Design review of the part built by this model. Coordinates are the model's own, in mm. A direction names the side the tool comes from. Round coordinates to 2 decimals unless told otherwise and drop trailing zeros. Order: outer loops, then holes, each group sorted by start corner. A loop starts at its lowest first (then second) coordinate and runs counter-clockwise, first axis right, second up. Notation, with made-up numbers: (29, 78) - (76, 78) arc R18 cw to (76, 88) - close; hole circle Ø8 at (22, 80). An arc over 180 degrees is marked (long way). Write item = value, one per line.
from build123d import *

# Parameters (mm, degrees)
SKETCH_1_R          = 12.25
SKETCH_1_R_2        = 5.5
SKETCH_1_R_3        = 1.25
EXTRUDE_1_DEPTH     = 3.5
SKETCH_2_R          = 2.25
CUT_EXTRUDE_1_DEPTH = 2
CHAMFER_1_SIZE      = 1


with BuildPart() as part:
    # Эскиз1 → Бобышка-Вытянуть1 (new body)
    with BuildSketch(Plane(origin=(0, 0, 0), x_dir=(1, 0, 0), z_dir=(0, 1, 0))):
        with Locations(Location((0, 0, 0), (0, 0, 270))):
            Circle(SKETCH_1_R)
        with Locations(Location((0, 0, 0), (0, 0, 270))):
            Circle(SKETCH_1_R_2, mode=Mode.SUBTRACT)
        with Locations(Location((0, 9.5, 0), (0, 0, 270))):
            Circle(SKETCH_1_R_3, mode=Mode.SUBTRACT)
        with Locations(Location((9.5, 0, 0), (0, 0, 270))):
            Circle(SKETCH_1_R_3, mode=Mode.SUBTRACT)
        with Locations(Location((0, -9.5, 0), (0, 0, 270))):
            Circle(SKETCH_1_R_3, mode=Mode.SUBTRACT)
        with Locations(Location((-9.5, 0, 0), (0, 0, 270))):
            Circle(SKETCH_1_R_3, mode=Mode.SUBTRACT)
    extrude(amount=EXTRUDE_1_DEPTH)

    # Эскиз2 → Вырез-Вытянуть1 (cut)
    with BuildSketch(Plane(origin=(0, 3.5, 0), x_dir=(1, 0, 0), z_dir=(0, 1, 0))):
        with Locations(Location((0, 9.5, 0), (0, 0, 270))):
            Circle(SKETCH_2_R)
        with Locations(Location((9.5, 0, 0), (0, 0, 270))):
            Circle(SKETCH_2_R)
        with Locations(Location((0, -9.5, 0), (0, 0, 270))):
            Circle(SKETCH_2_R)
        with Locations(Location((-9.5, 0, 0), (0, 0, 270))):
            Circle(SKETCH_2_R)
    extrude(amount=-CUT_EXTRUDE_1_DEPTH, mode=Mode.SUBTRACT)

    # Фаска1
    chamfer_1_edges = [part.edges().sort_by_distance(p)[0] for p in [
        (0, 3.5, -5.5),
    ]]
    chamfer(chamfer_1_edges, length=CHAMFER_1_SIZE)


solid = part.part
1) The part is to be moulded in two halves that separate along Z. For faces 3 (the cylindrical face through (10.74, 0.74, -0.16)), 4 (the cylindrical face through (3.68, 1.726, 11.684)), 5 (the flat face through (0, 0, -6)), say which applies: released by +Z, released by -Z, zero draft, split by the parting line, or undercut.
Findings:
face_3 = undercut
face_4 = split by the parting line
face_5 = zero draft
2) We need section A-A on x = 0. Write out the cut boundary in (y, z).
Findings:
outline = (0, -12.25) - (3.5, -12.25) - (3.5, -11.75) - (1.5, -11.75) - (1.5, -10.75) - (0, -10.75) - close; (0, -8.25) - (1.5, -8.25) - (1.5, -7.25) - (3.5, -7.25) - (3.5, -6.5) - (2.5, -5.5) - (0, -5.5) - close; (0, 5.5) - (2.5, 5.5) - (3.5, 6.5) - (3.5, 7.25) - (1.5, 7.25) - (1.5, 8.25) - (0, 8.25) - close; (0, 10.75) - (1.5, 10.75) - (1.5, 11.75) - (3.5, 11.75) - (3.5, 12.25) - (0, 12.25) - close
3) For faces 1 (the cylindrical face through (11.73, 2.51, -0.29)), 2 (the flat face through (-5, 3.5, 5)), list the 3-axis set-ups (+Z, -Z, +X, -X, +Y, -Y) from which the entire face can be reached by the end or side of a thin tool; tool diameter is ignored.
Findings:
face_1 = +Y
face_2 = +Z, -Z, +X, -X, +Y
4) We need section C-C on y = 1.85. Write out the cut boundary in (x, z).
Findings:
outline = circle Ø24.5 at (0, 0); hole circle Ø4.5 at (-9.5, 0); hole circle Ø11 at (0, 0); hole circle Ø4.5 at (0, -9.5); hole circle Ø4.5 at (0, 9.5); hole circle Ø4.5 at (9.5, 0)
5) Clearance check with flat-ended pins moving along their axes: pin 1 Ø4 at (x, z) = (0, 9.5) entering from +Y; pin 2 Ø1 at (y, z) = (3, 1.5) entering from +X; pin 3 Ø1 at (x, y) = (8.5, 3) entering from -Z. State where each tip first meets the part, or that it passes through.
Findings:
pin_1 = 1.5
pin_2 = 12.21
pin_3 = -9.28
6) We need section B-B on z = 8.75. Write out the cut boundary in (x, y), and give its area (3 significant figures).
Findings:
outline = (-8.57, 0) - (-1, 0) - (-1, 1.5) - (-2.12, 1.5) - (-2.12, 3.5) - (-8.57, 3.5) - close; (1, 0) - (8.57, 0) - (8.57, 3.5) - (2.12, 3.5) - (2.12, 1.5) - (1, 1.5) - close
area = 48.5 mm^2
7) To check wall thickness, follow L1, parallel to X at y = 0.4, z = 0; L2, parallel to X at y = 3.35, z = 1; L3, parallel to Z at x = 1.5, y = 2.35. State the ranges of each line that lie inside material, in increasing order. Write a range as from..to.
Findings:
L1 = -12.25..-10.75, -8.25..-5.5, 5.5..8.25, 10.75..12.25
L2 = -12.21..-11.52, -7.48..-6.27, 6.27..7.48, 11.52..12.21
L3 = -12.16..-11.18, -7.82..-5.29, 5.29..7.82, 11.18..12.16
8) We need section D-D on z = 0. Write out the cut boundary in (x, y).
Findings:
outline = (-12.25, 0) - (-10.75, 0) - (-10.75, 1.5) - (-11.75, 1.5) - (-11.75, 3.5) - (-12.25, 3.5) - close; (-8.25, 0) - (-5.5, 0) - (-5.5, 2.5) - (-6.5, 3.5) - (-7.25, 3.5) - (-7.25, 1.5) - (-8.25, 1.5) - close; (5.5, 0) - (8.25, 0) - (8.25, 1.5) - (7.25, 1.5) - (7.25, 3.5) - (6.5, 3.5) - (5.5, 2.5) - close; (10.75, 0) - (12.25, 0) - (12.25, 3.5) - (11.75, 3.5) - (11.75, 1.5) - (10.75, 1.5) - close
